Work out the finished part from the listing and answer in its coordinate system (mm). A direction names the side the tool comes from. Give positions to 0.01 mm unless a question says otherwise; leave off trailing zeros. Loops run counter-clockwise (first coordinate to the right, second up) from the corner with the lowest first, then second, coordinate; pieces in that order, holes last. Notation, with made-up numbers: M 46.5,-8 L 62.5,-8 A14 ccw 62.5,14 Z; hole C -2,9.5 d3. An arc over 180 degrees is marked long. Use a Markdown table: item, result.
```python
from build123d import *

# Parameters (mm, degrees)
CROQUIS1_R              = 75
CROQUIS1_W              = 100
CROQUIS1_H              = 100
SALIENTE_EXTRUIR1_DEPTH = 15
REDONDEO1_R             = 10
BARRER1_OUTLINE_R       = 75
BARRER1_ANGLE           = 45
CROQUIS6_R              = 75
CROQUIS6_R_2            = 63
SALIENTE_EXTRUIR3_DEPTH = 15


# Read off the part's stored shape, not the designer's step: Barrer1
with BuildPart() as part:
    # Croquis1 → Saliente-Extruir1 (new body)
    with BuildSketch(Plane(origin=(0, 0, 0), x_dir=(1, 0, 0), z_dir=(0, 1, 0))):
        with Locations(Location((0, 0, 0), (0, 0, 270))):
            Circle(CROQUIS1_R)
        Rectangle(CROQUIS1_W, CROQUIS1_H, mode=Mode.SUBTRACT)
    extrude(amount=SALIENTE_EXTRUIR1_DEPTH)

    # Redondeo1
    redondeo1_edges = [part.edges().sort_by_distance(p)[0] for p in [
        (50, 7.5, 50),
        (50, 7.5, -50),
        (-50, 7.5, -50),
        (-50, 7.5, 50),
    ]]
    fillet(redondeo1_edges, radius=REDONDEO1_R)

    # Barrer1 outline → Barrer1 (revolve)
    with BuildSketch(Plane(origin=(0, 0, 120), x_dir=(0, -0.7071067811865493, -0.7071067811865457), z_dir=(0, -0.7071067811865457, 0.7071067811865493))):
        with Locations((120, 0)):
            Circle(BARRER1_OUTLINE_R)
        with BuildLine():
            Line((80, 50), (160, 50))
            ThreePointArc((160, 50), (167.071067812, 47.071067812), (170, 40))
            Line((170, 40), (170, -40))
            ThreePointArc((170, -40), (167.071067812, -47.071067812), (160, -50))
            Line((160, -50), (80, -50))
            ThreePointArc((80, -50), (72.928932188, -47.071067812), (70, -40))
            Line((70, -40), (70, 40))
            ThreePointArc((70, 40), (72.928932188, 47.071067812), (80, 50))
        make_face(mode=Mode.SUBTRACT)
    revolve(axis=Axis((0, 0, 120), (1, 0, 0)), revolution_arc=BARRER1_ANGLE)

    # Croquis6 → Saliente-Extruir3 (add)
    with BuildSketch(Plane(origin=(0, -60, 60), x_dir=(1, 0, 0), z_dir=(0, -0.7071067811865467, 0.7071067811865485))):
        with Locations(Location((0, -35.147186258, 0), (0, 0, 270))):
            Circle(CROQUIS6_R)
        with Locations(Location((0, -35.147186258, 0), (0, 0, 52.528004817))):
            Circle(CROQUIS6_R_2, mode=Mode.SUBTRACT)
    extrude(amount=SALIENTE_EXTRUIR3_DEPTH)


solid = part.part
```
(1) A cutting plane is placed at C-C (x = 0). Write down the section's boundary in (y, z), and give its area (3 significant figures).
Entries:
| item | result |
|---|---|
| outline | M -148.49,-7.28 L -137.89,-17.89 A195 ccw 0,-75 L 15,-75 L 15,-50 L 0,-50 A170 cw -120.21,-0.21 L -129.4,-9.4 L -140.01,1.21 Z; M -50.91,90.3 L -40.31,79.69 L -49.5,70.5 A70 ccw 0,50 L 15,50 L 15,75 L 0,75 A45 cw -31.82,88.18 L -42.43,98.79 Z |
| area | 5,820 mm² |
(2) Consider probe 1 along Z at (x, y) = (6, -44); probe 2 along X at (y, z) = (-55, 60.5); probe 3 along X at (y, z) = (-32, -6). Determine where each line is inside the solid, lowest interval first. Write a range as [from, to].
Entries:
| item | result |
|---|---|
| probe 1 | z = [-69.72, -44.21], [65.56, 76], [82.98, 97.21] |
| probe 2 | x = [-64.08, -50], [50, 64.08] |
| probe 3 | x = [-74.33, -50], [50, 74.33] |
(3) A cutting plane is placed at B-B (x = 32.5). Write down the section's boundary in (y, z).
Entries:
| item | result |
|---|---|
| outline | M -143.25,-2.04 L -132.65,-12.65 A187.59 ccw 0,-67.59 L 15,-67.59 L 15,-50 L 0,-50 A170 cw -120.21,-0.21 L -123.02,-3.02 L -133.62,7.59 Z; M -57.3,83.92 L -46.69,73.31 L -49.5,70.5 A70 ccw 0,50 L 15,50 L 15,67.59 L 0,67.59 A52.41 cw -37.06,82.94 L -47.66,93.55 Z |
(4) Given P1, Ø4, axis at x = 19.5, y = -61.5, coming from the -Z side; P2, Ø1, axis at y = -18, z = -17, coming from the +X side; P3, Ø2, axis at x = 19.5, y = -84, coming from the -Z side, each flat-ended and moving along its own axis, determine where each tip first touches the part or whether it passes through.
Entries:
| item | result |
|---|---|
| P1 | stops at z = -63.19 |
| P2 | stops at x = 72.89 |
| P3 | stops at z = -53.68 |
(5) The mould has two halves that part along Y. Classify faces 1 (the flat face through (1, -46, 74)), 2 (the flat face through (1, -124, -4)), 3 (the flat face through (-1, 7, -50)), 4 (the flat face through (-46, -53, 67)): released by +Y, released by -Y, zero draft, split by the parting line, or undercut.
Entries:
| item | result |
|---|---|
| face 1 | released by -Y |
| face 2 | undercut |
| face 3 | zero draft |
| face 4 | undercut |
(6) Which of the six approach directions +Z, -Z, +X, -X, +Y, -Y give full straight-line access (tool end or side, diameter ignored) to faces 5 (the flat face through (-55, -84, 36)), 6 (the flat face through (61.461, -83.427, 57.786)), 7 (the flat face through (-1, 7, 50)), 8 (the cylindrical face through (-46.99, 7.6, -47.15)), 9 (the flat face through (51, 15, -1))?
Entries:
| item | result |
|---|---|
| face 5 | none |
| face 6 | +Z, +X, -X, -Y |
| face 7 | +Y, -Y |
| face 8 | +Y |
| face 9 | +Z, -Z, +X, -X, +Y |
(7) A cutting plane is placed at A-A (y = 4). Write down the section's boundary in (x, z).
Entries:
| item | result |
|---|---|
| outline | C 0,0 d150; hole M -50,-40 A10 ccw -40,-50 L 40,-50 A10 ccw 50,-40 L 50,40 A10 ccw 40,50 L -40,50 A10 ccw -50,40 Z |
